from build123d import *

# Parameters (mm, degrees)
FILLET_1_R = 1.5


with BuildPart() as part:
    # 草图1 → 旋转2 (revolve)
    with BuildSketch(Plane.XY, mode=Mode.PRIVATE) as revolve_2_sk:
        Polygon((-12.155060406, 4), (-5.915060406, 4), (-5.915060406, 6), (-7.535060406, 6), (-7.535060406, 15), (-10.535060406, 15), (-10.535060406, 6), (-12.155060406, 6), align=None)
    revolve(revolve_2_sk.sketch.rotate(Axis((-24.331674281, 0, 0), (1, 0, 0)), 90), axis=Axis((-24.331674281, 0, 0), (1, 0, 0)))

    # 圆角1
    fillet_1_edges = [part.edges().sort_by_distance(p)[0] for p in [
        (-10.535060406, 0, -15),
        (-7.535060406, 0, -15),
    ]]
    fillet(fillet_1_edges, radius=FILLET_1_R - 0.0001)  # a hair under: the kernel refuses the full size


solid = part.part
For this review, take the finished solid that the model builds, in its own axes (mm). A direction names the side the tool comes from. Round coordinates to 2 decimals unless told otherwise and drop trailing zeros. Order: outer loops, then holes, each group sorted by start corner. A loop starts at its lowest first (then second) coordinate and runs counter-clockwise, first axis right, second up. Notation, with made-up numbers: (28, 4) -> (70, 4) arc R17 ccw to (70, 18) -> close; hole circle Ø1 at (51.25, -25.75). An arc over 180 degrees is marked (long way). Write item = value, one per line. Start each with the question number.
1) Take a section at D-D on x = -8. State the section outline as (y, z) points, plus the area to 3 significant figures.
2) Tool access review of faces 1 (the face through (-7.535, 3, -6)), 2 (the face through (-11.356, -1.802, 5.723)), 3 (the face through (-5.915, 3.92, 1.42)): name each direction out of +Z, -Z, +X, -X, +Y, -Y from which nothing blocks a thin tool from reaching the whole face with its end or side.
3) Take a section at C-C on x = -11. State the section outline as (y, z) points.
4) To check wall thickness, follow line 1 (Y direction, x = -10.75, z = 0); line 2 (X direction, y = 4.5, z = 12.5); line 3 (Y direction, x = -8.5, z = 0.75). State the ranges of each line that lie inside material, in increasing order. Write a range as from..to.
5) Insertion check: pin 1 (2 mm diameter, centred on x = -7, z = 7.5, fed in from +Y); pin 2 (10 mm diameter, centred on y = -10.5, z = 12, fed in from -X); pin 3 (2 mm diameter, centred on x = -7, z = 9.5, fed in from -Y). Each pin has a flat end and moves straight along its axis. Give the tip position at first contact, or say it passes through.
6) The part is to be moulded in two halves that separate along Y. For faces 4 (the face through (-10.535, 6, 3)), 5 (the face through (-8.991, 3.905, -0.867)), 6 (the face through (-6.736, -1.802, 5.723)), say which applies: +Y half, -Y half, draft (parallel to the pull), parting line (faces both ways), or undercut.
Verdict:
q1.outline = circle Ø29.17 at (0, 0); hole circle Ø8 at (0, 0)
q1.area = 618 mm2
q2.face_1 = +X
q2.face_2 = -X
q2.face_3 = +Z, -Z, +X, +Y, -Y
q3.outline = circle Ø12 at (0, 0); hole circle Ø8 at (0, 0)
q4.line_1 = -6..-4, 4..6
q4.line_2 = -10.54..-7.54
q4.line_3 = -14.88..-3.93, 3.93..14.88
q5.pin_1 = 12.64
q5.pin_2 = -10.54
q5.pin_3 = -11.29
q6.face_4 = draft
q6.face_5 = undercut
q6.face_6 = parting line
